```python
from build123d import *

# Parameters (mm, degrees)
SKETCH1_R                        = 9.5
SKETCH1_W                        = 55
SKETCH1_H                        = 123
FOND_DEPTH                       = 4
TROUS_STEPPERS_REACH             = 157.615
SKETCH5_R                        = 1.5
SKETCH5_R_2                      = 2.75
TROUS_STEPPERS_DIRECTION_2_DEPTH = 156.614909311
TROUS_POULIES_REACH              = 157.615
SKETCH7_R                        = 2
TROUS_CARTE_REACH                = 157.615
SKETCH9_R                        = 1.5


with BuildPart() as part:
    # Sketch1 → fond (new body)
    with BuildSketch(Plane(origin=(0, 0, 0), x_dir=(1, 0, 0), z_dir=(0, 1, 0))):
        with BuildLine():
            ThreePointArc((-110, 0), (0, 110), (110, 0))
            ThreePointArc((110, 0), (90.069417673, -63.146654702), (37.5, -103.4105894))
            ThreePointArc((37.5, -103.4105894), (0, -110), (-37.5, -103.4105894))
            ThreePointArc((-37.5, -103.4105894), (-90.069417673, -63.146654702), (-110, 0))
        make_face()
        with Locations(Location((0, 96, 0), (0, 0, 270))):
            Circle(SKETCH1_R, mode=Mode.SUBTRACT)
        with Locations((0, -15.5)):
            Rectangle(SKETCH1_W, SKETCH1_H, mode=Mode.SUBTRACT)
    extrude(amount=FOND_DEPTH)

    # Sketch5 → trous steppers (cut, up to next)
    with BuildSketch(Plane(origin=(0, 4, 0), x_dir=(1, 0, 0), z_dir=(0, 1, 0)), mode=Mode.PRIVATE) as trous_steppers_sk1:
        with Locations(Location((36.787473029, 56.456130336, 0), (0, 0, 90))):
            Circle(SKETCH5_R)
    trous_steppers_tool1 = extrude(trous_steppers_sk1.sketch, amount=-TROUS_STEPPERS_REACH, mode=Mode.PRIVATE) & part.part
    # Sketch5 → trous steppers (cut, up to next)
    with BuildSketch(Plane(origin=(0, 4, 0), x_dir=(1, 0, 0), z_dir=(0, 1, 0)), mode=Mode.PRIVATE) as trous_steppers_sk2:
        with Locations(Location((58.707783245, 78.376440552, 0), (0, 0, 90))):
            Circle(SKETCH5_R)
    trous_steppers_tool2 = extrude(trous_steppers_sk2.sketch, amount=-TROUS_STEPPERS_REACH, mode=Mode.PRIVATE) & part.part
    # Sketch5 → trous steppers (cut, up to next)
    with BuildSketch(Plane(origin=(0, 4, 0), x_dir=(1, 0, 0), z_dir=(0, 1, 0)), mode=Mode.PRIVATE) as trous_steppers_sk3:
        with Locations(Location((80.628093462, 56.456130336, 0), (0, 0, 90))):
            Circle(SKETCH5_R)
    trous_steppers_tool3 = extrude(trous_steppers_sk3.sketch, amount=-TROUS_STEPPERS_REACH, mode=Mode.PRIVATE) & part.part
    # Sketch5 → trous steppers (cut, up to next)
    with BuildSketch(Plane(origin=(0, 4, 0), x_dir=(1, 0, 0), z_dir=(0, 1, 0)), mode=Mode.PRIVATE) as trous_steppers_sk4:
        with Locations(Location((-80.628093462, 56.456130336, 0), (0, 0, 90))):
            Circle(SKETCH5_R)
    trous_steppers_tool4 = extrude(trous_steppers_sk4.sketch, amount=-TROUS_STEPPERS_REACH, mode=Mode.PRIVATE) & part.part
    # Sketch5 → trous steppers (cut, up to next)
    with BuildSketch(Plane(origin=(0, 4, 0), x_dir=(1, 0, 0), z_dir=(0, 1, 0)), mode=Mode.PRIVATE) as trous_steppers_sk5:
        with Locations(Location((-58.707783245, 78.376440552, 0), (0, 0, 90))):
            Circle(SKETCH5_R)
    trous_steppers_tool5 = extrude(trous_steppers_sk5.sketch, amount=-TROUS_STEPPERS_REACH, mode=Mode.PRIVATE) & part.part
    # Sketch5 → trous steppers (cut, up to next)
    with BuildSketch(Plane(origin=(0, 4, 0), x_dir=(1, 0, 0), z_dir=(0, 1, 0)), mode=Mode.PRIVATE) as trous_steppers_sk6:
        with Locations(Location((-36.787473029, 56.456130336, 0), (0, 0, 90))):
            Circle(SKETCH5_R)
    trous_steppers_tool6 = extrude(trous_steppers_sk6.sketch, amount=-TROUS_STEPPERS_REACH, mode=Mode.PRIVATE) & part.part
    # Sketch5 → trous steppers (cut, up to next)
    with BuildSketch(Plane(origin=(0, 4, 0), x_dir=(1, 0, 0), z_dir=(0, 1, 0)), mode=Mode.PRIVATE) as trous_steppers_sk7:
        with Locations(Location((58.707783245, 56.456130336, 0), (0, 0, 90))):
            Circle(SKETCH5_R_2)
    trous_steppers_tool7 = extrude(trous_steppers_sk7.sketch, amount=-TROUS_STEPPERS_REACH, mode=Mode.PRIVATE) & part.part
    # Sketch5 → trous steppers (cut, up to next)
    with BuildSketch(Plane(origin=(0, 4, 0), x_dir=(1, 0, 0), z_dir=(0, 1, 0)), mode=Mode.PRIVATE) as trous_steppers_sk8:
        with Locations(Location((-58.707783245, 56.456130336, 0), (0, 0, 90))):
            Circle(SKETCH5_R_2)
    trous_steppers_tool8 = extrude(trous_steppers_sk8.sketch, amount=-TROUS_STEPPERS_REACH, mode=Mode.PRIVATE) & part.part
    add(trous_steppers_tool1.solids().sort_by_distance((36.787473, 4, -56.45613))[0], mode=Mode.SUBTRACT)
    add(trous_steppers_tool2.solids().sort_by_distance((58.707783, 4, -78.376441))[0], mode=Mode.SUBTRACT)
    add(trous_steppers_tool3.solids().sort_by_distance((80.628093, 4, -56.45613))[0], mode=Mode.SUBTRACT)
    add(trous_steppers_tool4.solids().sort_by_distance((-80.628093, 4, -56.45613))[0], mode=Mode.SUBTRACT)
    add(trous_steppers_tool5.solids().sort_by_distance((-58.707783, 4, -78.376441))[0], mode=Mode.SUBTRACT)
    add(trous_steppers_tool6.solids().sort_by_distance((-36.787473, 4, -56.45613))[0], mode=Mode.SUBTRACT)
    add(trous_steppers_tool7.solids().sort_by_distance((58.707783, 4, -56.45613))[0], mode=Mode.SUBTRACT)
    add(trous_steppers_tool8.solids().sort_by_distance((-58.707783, 4, -56.45613))[0], mode=Mode.SUBTRACT)

    # Sketch5 → trous steppers direction 2 (cut)
    with BuildSketch(Plane(origin=(0, 4, 0), x_dir=(1, 0, 0), z_dir=(0, 1, 0))):
        with Locations(Location((36.787473029, 56.456130336, 0), (0, 0, 90))):
            Circle(SKETCH5_R)
        with Locations(Location((58.707783245, 78.376440552, 0), (0, 0, 90))):
            Circle(SKETCH5_R)
        with Locations(Location((80.628093462, 56.456130336, 0), (0, 0, 90))):
            Circle(SKETCH5_R)
        with Locations(Location((-80.628093462, 56.456130336, 0), (0, 0, 90))):
            Circle(SKETCH5_R)
        with Locations(Location((-58.707783245, 78.376440552, 0), (0, 0, 90))):
            Circle(SKETCH5_R)
        with Locations(Location((-36.787473029, 56.456130336, 0), (0, 0, 90))):
            Circle(SKETCH5_R)
        with Locations(Location((58.707783245, 56.456130336, 0), (0, 0, 90))):
            Circle(SKETCH5_R_2)
        with Locations(Location((-58.707783245, 56.456130336, 0), (0, 0, 90))):
            Circle(SKETCH5_R_2)
    extrude(amount=TROUS_STEPPERS_DIRECTION_2_DEPTH, mode=Mode.SUBTRACT)

    # Sketch7 → trous poulies (cut, up to next)
    with BuildSketch(Plane(origin=(0, 4, 0), x_dir=(1, 0, 0), z_dir=(0, 1, 0)), mode=Mode.PRIVATE) as trous_poulies_sk1:
        with Locations(Location((80.628093462, 35.675463443, 0), (0, 0, 270))):
            Circle(SKETCH7_R)
    trous_poulies_tool1 = extrude(trous_poulies_sk1.sketch, amount=-TROUS_POULIES_REACH, mode=Mode.PRIVATE) & part.part
    # Sketch7 → trous poulies (cut, up to next)
    with BuildSketch(Plane(origin=(0, 4, 0), x_dir=(1, 0, 0), z_dir=(0, 1, 0)), mode=Mode.PRIVATE) as trous_poulies_sk2:
        with Locations(Location((-80.628093462, 35.675463443, 0), (0, 0, 90))):
            Circle(SKETCH7_R)
    trous_poulies_tool2 = extrude(trous_poulies_sk2.sketch, amount=-TROUS_POULIES_REACH, mode=Mode.PRIVATE) & part.part
    add(trous_poulies_tool1.solids().sort_by_distance((80.628093, 4, -35.675463))[0], mode=Mode.SUBTRACT)
    add(trous_poulies_tool2.solids().sort_by_distance((-80.628093, 4, -35.675463))[0], mode=Mode.SUBTRACT)

    # Sketch9 → trous carte (cut, up to next)
    with BuildSketch(Plane(origin=(0, 4, 0), x_dir=(1, 0, 0), z_dir=(0, 1, 0)), mode=Mode.PRIVATE) as trous_carte_sk1:
        with Locations(Location((-49.687242847, 18.164395088, 0), (0, 0, 270))):
            Circle(SKETCH9_R)
    trous_carte_tool1 = extrude(trous_carte_sk1.sketch, amount=-TROUS_CARTE_REACH, mode=Mode.PRIVATE) & part.part
    # Sketch9 → trous carte (cut, up to next)
    with BuildSketch(Plane(origin=(0, 4, 0), x_dir=(1, 0, 0), z_dir=(0, 1, 0)), mode=Mode.PRIVATE) as trous_carte_sk2:
        with Locations(Location((-77.887242847, 18.164395088, 0), (0, 0, 270))):
            Circle(SKETCH9_R)
    trous_carte_tool2 = extrude(trous_carte_sk2.sketch, amount=-TROUS_CARTE_REACH, mode=Mode.PRIVATE) & part.part
    # Sketch9 → trous carte (cut, up to next)
    with BuildSketch(Plane(origin=(0, 4, 0), x_dir=(1, 0, 0), z_dir=(0, 1, 0)), mode=Mode.PRIVATE) as trous_carte_sk3:
        with Locations(Location((-93.187242847, -38.350487124, 0), (0, 0, 270))):
            Circle(SKETCH9_R)
    trous_carte_tool3 = extrude(trous_carte_sk3.sketch, amount=-TROUS_CARTE_REACH, mode=Mode.PRIVATE) & part.part
    # Sketch9 → trous carte (cut, up to next)
    with BuildSketch(Plane(origin=(0, 4, 0), x_dir=(1, 0, 0), z_dir=(0, 1, 0)), mode=Mode.PRIVATE) as trous_carte_sk4:
        with Locations(Location((-45.087242847, -38.350487124, 0), (0, 0, 270))):
            Circle(SKETCH9_R)
    trous_carte_tool4 = extrude(trous_carte_sk4.sketch, amount=-TROUS_CARTE_REACH, mode=Mode.PRIVATE) & part.part
    add(trous_carte_tool1.solids().sort_by_distance((-49.687243, 4, -18.164395))[0], mode=Mode.SUBTRACT)
    add(trous_carte_tool2.solids().sort_by_distance((-77.887243, 4, -18.164395))[0], mode=Mode.SUBTRACT)
    add(trous_carte_tool3.solids().sort_by_distance((-93.187243, 4, 38.350487))[0], mode=Mode.SUBTRACT)
    add(trous_carte_tool4.solids().sort_by_distance((-45.087243, 4, 38.350487))[0], mode=Mode.SUBTRACT)


solid = part.part
```
Check sheet for the modelled part. Datum: model origin and axes. Units: mm. Round coordinates to 2 decimals unless told otherwise and drop trailing zeros. Loops run counter-clockwise (first coordinate to the right, second up) from the corner with the lowest first, then second, coordinate; pieces in that order, holes last. Notation, with made-up numbers: (-7.5, 24.5) - (22.5, 24.5) arc R25 cw to (22.5, 60.5) - close; hole circle Ø4 at (-14, 65.5). An arc over 180 degrees is marked (long way). Write item = value, one per line. Start each with the question number.
Q1. Release check for a two-part mould opening along X. For faces 1 (the face through (56.85, 2.03, -54.43)), 2 (the face through (-47, 4, -2)) record: pulls with the +X half, pulls with the -X half, needs draft (parallel to the pull), parting line crosses it, or undercut.
Q2. Section check A-A (x = 0). Record the boundary of the cut face in (y, z).
Q3. Section check B-B (z = -96). Record the boundary of the cut face in (x, y), plus the area to 3 significant figures.
Q4. Section check D-D (z = 44.5). Record the boundary of the cut face in (x, y), plus the area to 3 significant figures.
Q5. Section check C-C (y = 0.6). Count the separate pieces of the cut face and the enclosed holes in it, plus the area to 3 significant figures.
Q6. Depth check by flat-ended pin: P1, Ø10, axis at x = -68, z = -87, coming from the -Y side; P2, Ø2, axis at x = 28.5, y = 0.5, coming from the -Z side. Enter the tip coordinate at first touch or a pass-through.
Q7. Thickness scan on L1, parallel to Z at x = 1, y = 3.5; L2, parallel to Z at x = 2, y = 0.8; L3, parallel to X at y = 1, z = -96. Record the ranges inside material, lowest first.
Derived:
q1.face_1 = undercut
q1.face_2 = needs draft
q2.outline = (0, -110) - (4, -110) - (4, -105.5) - (0, -105.5) - close; (0, -86.5) - (4, -86.5) - (4, -46) - (0, -46) - close; (0, 77) - (4, 77) - (4, 110) - (0, 110) - close
q3.outline = (-53.7, 0) - (-9.5, 0) - (-9.5, 4) - (-53.7, 4) - close; (9.5, 0) - (53.7, 0) - (53.7, 4) - (9.5, 4) - close
q3.area = 354 mm^2
q4.outline = (-100.6, 0) - (-27.5, 0) - (-27.5, 4) - (-100.6, 4) - close; (27.5, 0) - (100.6, 0) - (100.6, 4) - (27.5, 4) - close
q4.area = 585 mm^2
q5.separate_pieces = 1
q5.enclosed_holes = 16
q5.area = 30,800 mm^2
q6.P1 = 0
q6.P2 = -106.51
q7.L1 = -110 to -105.45, -86.55 to -46, 77 to 110
q7.L2 = -109.98 to -105.29, -86.71 to -46, 77 to 109.98
q7.L3 = -53.7 to -9.5, 9.5 to 53.7
